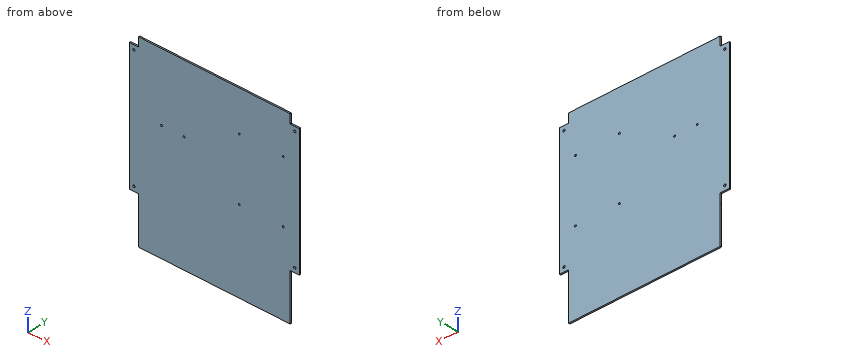
from build123d import *

# Parameters (mm, degrees)
BOSS_EXTRUDE1_DEPTH = 3.175
SKETCH4_R           = 2
CUT_EXTRUDE2_DEPTH  = 3.175
SKETCH7_W           = 20
SKETCH7_H           = 389.675
CUT_EXTRUDE6_DEPTH  = 3.175
SKETCH8_W           = 20.01
SKETCH8_H           = 84
SKETCH8_W_2         = 20.1
SKETCH8_H_2         = 84.09
CUT_EXTRUDE7_DEPTH  = 3.175
SKETCH9_R           = 2.5
CUT_EXTRUDE8_DEPTH  = 3.175


with BuildPart() as part:
    # Sketch1 → Boss-Extrude1 (new body)
    with BuildSketch(Plane(origin=(0, 0, 0), x_dir=(1, 0, 0), z_dir=(0, 1, 0))):
        Polygon((-165.06435994, -204.65564006), (-165.06435994, -184.65564006), (-204.97435994, -184.65564006), (-204.97435994, 100.92935994), (-165.06435994, 100.92935994), (-164.96435994, 121.01935994), (-204.97435994, 121.01935994), (-204.97435994, 205.01935994), (204.61064006, 205.01935994), (204.61064006, 121.01935994), (164.51064006, 120.92935994), (164.51064006, 100.92935994), (204.61064006, 100.92935994), (202.86064006, -184.65564006), (164.51064006, -184.65564006), (164.51064006, -204.65564006), align=None)
    extrude(amount=BOSS_EXTRUDE1_DEPTH)

    # Sketch4 → Cut-Extrude2 (cut)
    with BuildSketch(Plane(origin=(0, 3.175, 0), x_dir=(1, 0, 0), z_dir=(0, 1, 0))):
        with Locations(Location((-114.989359939, -54.80564006, 0), (0, 0, 270))):
            Circle(SKETCH4_R)
        with Locations(Location((-65.989359939, -54.80564006, 0), (0, 0, 270))):
            Circle(SKETCH4_R)
        with Locations(Location((54.010640061, -114.65564006, 0), (0, 0, 270))):
            Circle(SKETCH4_R)
        with Locations(Location((149.510640061, -114.65564006, 0), (0, 0, 270))):
            Circle(SKETCH4_R)
        with Locations(Location((54.010640061, 22.34435994, 0), (0, 0, 270))):
            Circle(SKETCH4_R)
        with Locations(Location((149.510640061, 22.34435994, 0), (0, 0, 270))):
            Circle(SKETCH4_R)
    extrude(amount=-CUT_EXTRUDE2_DEPTH, mode=Mode.SUBTRACT)

    # Sketch7 → Cut-Extrude6 (cut)
    with BuildSketch(Plane(origin=(0, 3.175, 0), x_dir=(1, 0, 0), z_dir=(0, 1, 0))):
        with Locations((-194.97435994, 10.18185994)):
            Rectangle(SKETCH7_W, SKETCH7_H)
        Polygon((204.61064006, 205.01935994), (184.61064006, 205.01935994), (184.61064006, -184.65564006), (202.86064006, -184.65564006), align=None)
    extrude(amount=-CUT_EXTRUDE6_DEPTH, mode=Mode.SUBTRACT)


with BuildPart() as body_2:
    # of the pieces the cut leaves, the one that is kept (cut_extrude6_keep)
    add(part.part.solids().sort_by_distance((-165.06435994, 0, 204.65564006))[0])

    # Sketch8 → Cut-Extrude7 (cut)
    with BuildSketch(Plane(origin=(0, 3.175, 0), x_dir=(1, 0, 0), z_dir=(0, 1, 0))):
        with Locations((-174.96935994, 163.01935994)):
            Rectangle(SKETCH8_W, SKETCH8_H)
        with Locations((174.56064006, 162.97435994)):
            Rectangle(SKETCH8_W_2, SKETCH8_H_2)
    extrude(amount=-CUT_EXTRUDE7_DEPTH, mode=Mode.SUBTRACT)

    # Sketch9 → Cut-Extrude8 (cut)
    with BuildSketch(Plane(origin=(0, 3.175, 0), x_dir=(1, 0, 0), z_dir=(0, 1, 0))):
        with Locations(Location((-175.01935994, -174.65564006, 0), (0, 0, 270))):
            Circle(SKETCH9_R)
        with Locations(Location((174.56064006, -174.65564006, 0), (0, 0, 270))):
            Circle(SKETCH9_R)
        with Locations(Location((174.56064006, 90.93435994, 0), (0, 0, 270))):
            Circle(SKETCH9_R)
        with Locations(Location((-175.01935994, 90.93435994, 0), (0, 0, 270))):
            Circle(SKETCH9_R)
    extrude(amount=-CUT_EXTRUDE8_DEPTH, mode=Mode.SUBTRACT)


solid = body_2.part
Geometry check sheet. Reference: the model listing, model coordinates, mm. Coordinates: 2 decimals unless noted, no trailing zeros. Order: outer loops, then holes, each group sorted by start corner. A loop starts at its lowest first (then second) coordinate and runs counter-clockwise, first axis right, second up. Notation, with made-up numbers: (13, -32.5) -> (50, -32.5) arc R29 ccw to (50, -7.5) -> close; hole circle Ø9 at (36.25, 28). An arc over 180 degrees is marked (long way). Use a Markdown table: item, result. Add a question column.
1. Cross-section at A-A (y = 2.4). Give the number of separate pieces and of enclosed holes in the cut face, and give its area (3 significant figures).
2. Material ranges on L1, parallel to X at y = 0.6, z = 53; L2, parallel to X at y = 2.75, z = -24; L3, parallel to Z at x = 165, y = 1.2, recorded low to high.
3. Cross-section at B-B (z = -152). Enter the section's corners in (x, y) (3 decimals).
4. Go/stop test with flat-tipped pins: pin 1 Ø1.6 at (y, z) = (1.5, -140.5) entering from +X; pin 2 Ø1.6 at (x, y) = (-172.5, 2) entering from -Z; pin 3 Ø1.6 at (y, z) = (1.5, -155.5) entering from -X. Record where each tip stops, or that it passes through.
Filled sheet:
| question | item | result |
|---|---|---|
| 1 | separate pieces | 1 |
| 1 | enclosed holes | 10 |
| 1 | area | 146,000 mm2 |
| 2 | L1 | -184.97 to -115.85, -114.13 to -66.85, -65.13 to 184.61 |
| 2 | L2 | -184.97 to 52.89, 55.13 to 148.39, 150.63 to 184.61 |
| 2 | L3 | -100.93 to 184.66 |
| 3 | outline | (-164.964, 0) -> (164.511, 0) -> (164.511, 3.175) -> (-164.964, 3.175) -> close |
| 4 | pin 1 | x = 164.51 |
| 4 | pin 2 | z = -100.93 |
| 4 | pin 3 | x = -164.96 |
